```python
from build123d import *

# Parameters (mm, degrees)
F0_W     = 120
F0_H     = 20
F1_DEPTH = 6
F2_R     = 1.575
F3_DEPTH = 6
F4_W     = 5
F4_H     = 20
F5_DEPTH = 6
F6_R     = 5


with BuildPart() as f1:
    # F0 (on Top) → F1 (new body)
    with BuildSketch(Plane.XY):
        Rectangle(F0_W, F0_H)
    extrude(amount=F1_DEPTH)

    # F2 (on face) → F3 (cut, through all)
    with BuildSketch(Plane.XY.offset(6)):
        with Locations((-53.1, 0)):
            Circle(F2_R)
        with Locations((-35.5, 0)):
            Circle(F2_R)
        with Locations((53.1, 0)):
            Circle(F2_R)
        with Locations((35.5, 0)):
            Circle(F2_R)
    extrude(amount=-F3_DEPTH, mode=Mode.SUBTRACT)

    # F4 (on Top) → F5 (join, through all)
    with BuildSketch(Plane.XY):
        with Locations((62.5, 0)):
            Rectangle(F4_W, F4_H)
    extrude(amount=F5_DEPTH)

    # F6
    f6_edges = [f1.edges().sort_by_distance(p)[0] for p in [
        (-60, -10, 3),
        (-60, 10, 3),
    ]]
    fillet(f6_edges, radius=F6_R)


solid = f1.part
```
Read the model definition and answer for the solid it produces. Units are mm, in the model's axes. Give positions to 0.01 mm unless a question says otherwise; leave off trailing zeros. Write each loop counter-clockwise with the first axis right and the second up, starting at its lowest first coordinate (ties: lowest second). Pieces come first, ordered by that corner, then holes. Notation, with made-up numbers: (69.25, -37) - (113.25, -37) arc R19 cw to (113.25, -10) - close; hole circle Ø3 at (-23.75, 28.25). An arc over 180 degrees is marked (long way). Write item = value, one per line. Start each with the question number.
Item 1: Find the intervals of material crossed by probe 1 along Y at (x, z) = (-35.5, 2.55) (3 decimals); probe 2 along X at (y, z) = (7.5, 5.75); probe 3 along Y at (x, z) = (36, 1.5), in increasing order. Write a range as [from, to].
Item 2: Find section A-A (y = 0). Give the vertices of the cut face in (x, z) (3 decimals), then the cut area to 3 significant figures.
Item 3: The mould has two halves that part along Y. Classify faces 1 (the flat face through (4, 10, 3)), 2 (the cylindrical face through (33.927, 0.069, 3.042)), 3 (the flat face through (65, 0, 3)): +Y half, -Y half, draft (parallel to the pull), parting line (faces both ways), or undercut.
Item 4: Find section C-C (z = 2.9). Give the vertices of the cut face in (x, y) (3 decimals).
Item 5: Find section B-B (x = -53.1). Give the vertices of the cut face in (y, z) (3 decimals), then the cut area to 3 significant figures.
Item 6: This flat-tipped pin is pushed along its axis until it touches: P1, Ø3.5, axis at x = -35.5, y = 0, coming from the -Z side. Where does it stop, or does it pass through?
Response:
q1.probe_1 = [-10, -1.575], [1.575, 10]
q1.probe_2 = [-59.33, 65]
q1.probe_3 = [-10, -1.49], [1.49, 10]
q2.outline = (-60, 0) - (-54.675, 0) - (-54.675, 6) - (-60, 6) - close; (-51.525, 0) - (-37.075, 0) - (-37.075, 6) - (-51.525, 6) - close; (-33.925, 0) - (33.925, 0) - (33.925, 6) - (-33.925, 6) - close; (37.075, 0) - (51.525, 0) - (51.525, 6) - (37.075, 6) - close; (54.675, 0) - (65, 0) - (65, 6) - (54.675, 6) - close
q2.area = 674 mm²
q3.face_1 = +Y half
q3.face_2 = undercut
q3.face_3 = draft
q4.outline = (-60, -5) arc R5 ccw to (-55, -10) - (65, -10) - (65, 10) - (-55, 10) arc R5 ccw to (-60, 5) - close; hole circle Ø3.15 at (-53.1, 0); hole circle Ø3.15 at (-35.5, 0); hole circle Ø3.15 at (35.5, 0); hole circle Ø3.15 at (53.1, 0)
q5.outline = (-10, 0) - (-1.575, 0) - (-1.575, 6) - (-10, 6) - close; (1.575, 0) - (10, 0) - (10, 6) - (1.575, 6) - close
q5.area = 101 mm²
q6.P1 = 0
